The drawing under review shows one solid part. Ordinate dimensions are in mm from its lowest x, y, z. A direction names the side the tool comes from. Coordinates: 2 decimals unless noted, no trailing zeros. Loops run counter-clockwise (first coordinate to the right, second up) from the corner with the lowest first, then second, coordinate; pieces in that order, holes last. Notation, with made-up numbers: M -23.5,88 L 11.5,88 A20 cw 11.5,100 Z; hole C -2.5,21.5 d3. An arc over 180 degrees is marked long. Put each result on its own line as item: value.
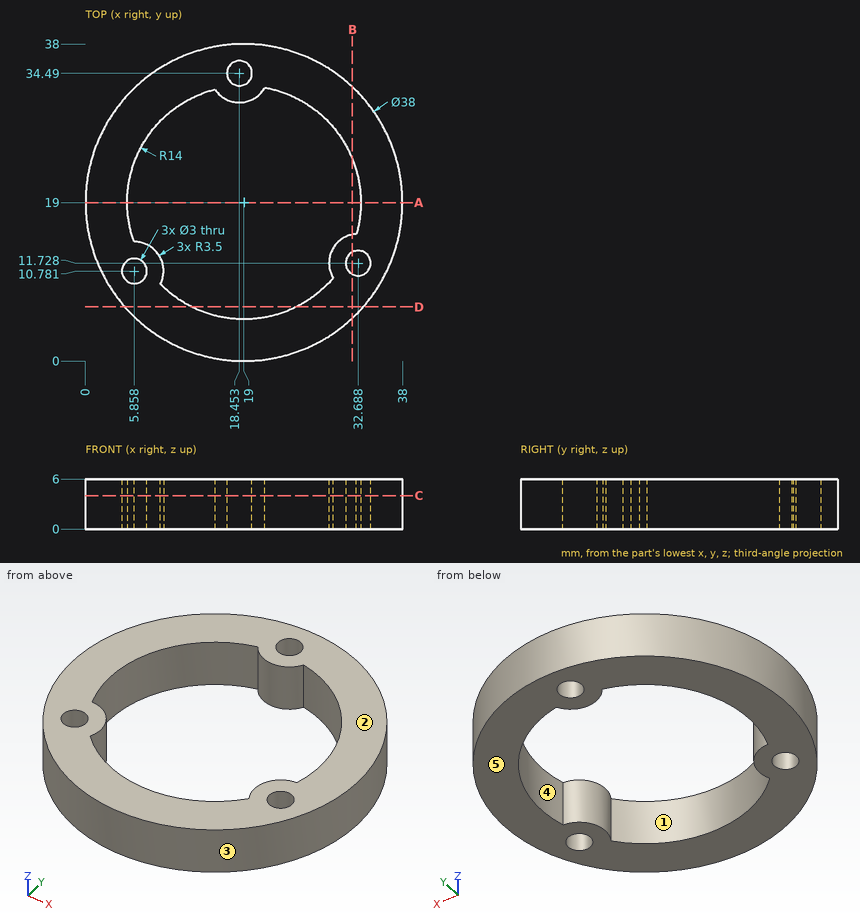
(1) Wall thickness on line 1 along X through (y, z) = (12.5, 1.4) (1 decimal); line 2 along X through (y, z) = (13, 0.4) (1 decimal); line 3 along Y through (x, z) = (26, 0.3) (1 decimal): over which ranges is each line inside the solid? List them lowest first. Write a range as [from, to].
Determined:
line 1: x = [1.1, 8.9], [29.3, 31.4], [34, 36.9]
line 2: x = [1, 8.6], [29.4, 31.9], [33.5, 37]
line 3: y = [1.3, 6.9], [31.1, 36.7]
(2) Add section C-C (z = 4). Write out the cut boundary in (x, y) (1 decimal).
Determined:
outline: C 19,19 d38; hole C 5.9,10.8 d3; hole M 5.8,14.3 A3.5 cw 9,9.2 A14 ccw 29.7,9.9 A3.5 cw 32.5,15.2 A14 ccw 21.5,32.8 A3.5 cw 15.5,32.6 A14 ccw Z; hole C 18.5,34.5 d3; hole C 32.7,11.7 d3
(3) Draft analysis for pull direction X (two halves, no side actions). For the marked faces 1, 2 and 3, state which applies: +X half, -X half, draft (parallel to the pull), parting line (faces both ways), or undercut.
Determined:
face 1: undercut
face 2: draft
face 3: parting line
(4) Tool access review of the marked faces 4 and 5: name each direction out of +Z, -Z, +X, -X, +Y, -Y from which nothing blocks a thin tool from reaching the whole face with its end or side.
Determined:
face 4: +Z, -Z
face 5: -Z, +X, -X, +Y, -Y
(5) Add section B-B (x = 32). Write out the cut boundary in (y, z) (1 decimal).
Determined:
outline: M 5.1,0 L 10.4,0 L 10.4,6 L 5.1,6 Z; M 13.1,0 L 15.2,0 L 15.2,6 L 13.1,6 Z; M 24.2,0 L 32.9,0 L 32.9,6 L 24.2,6 Z
(6) For pin 1 (12 mm diameter, centred on x = 9, y = 14.5, fed in from -Z); pin 2 (1 mm diameter, centred on x = 15, z = 4, fed in from +Y) (1 decimal); pin 3 (1 mm diameter, centred on y = 16.5, z = 5, fed in from +X); pin 4 (1.5 mm diameter, centred on x = 29, z = 4.5, fed in from -Y), all flat-tipped, find the tip position at first contact; note any pin that passes through.
Determined:
pin 1: stops at z = 0
pin 2: stops at y = 37.7
pin 3: stops at x = 37.89
pin 4: stops at y = 2.4
(7) Add section A-A (y = 19). Write out the cut boundary in (x, z), plus the area to 3 significant figures.
Determined:
outline: M 0,0 L 5,0 L 5,6 L 0,6 Z; M 33,0 L 38,0 L 38,6 L 33,6 Z
area: 60.0 mm^2
(8) Add section D-D (y = 6.5). Write out the cut boundary in (x, z) (1 decimal).
Determined:
outline: M 4.7,0 L 12.7,0 L 12.7,6 L 4.7,6 Z; M 25.3,0 L 33.3,0 L 33.3,6 L 25.3,6 Z
